Here's how the part is built. I have some questions about the finished solid (model axes, mm). Face numbers are marked on the shaded views. A direction names the side the tool comes from. Give positions to 0.01 mm unless a question says otherwise; leave off trailing zeros. Order: outer loops, then holes, each group sorted by start corner. A loop starts at its lowest first (then second) coordinate and runs counter-clockwise, first axis right, second up.
from build123d import *

# Parameters (mm, degrees)
SKETCH1_W           = 42
SKETCH1_H           = 42
BOSS_EXTRUDE1_DEPTH = 5
SKETCH2_R           = 1.65
CUT_EXTRUDE1_DEPTH  = 5
SKETCH3_W           = 5
SKETCH3_H           = 42
BOSS_EXTRUDE2_DEPTH = 10
SKETCH4_W           = 5
SKETCH4_H           = 10
BOSS_EXTRUDE3_DEPTH = 10
SKETCH5_R           = 1.65
CUT_EXTRUDE2_DEPTH  = 10
FILLET1_R           = 5
FILLET2_R           = 2
SKETCH6_R           = 11.5
CUT_EXTRUDE3_DEPTH  = 10


with BuildPart() as part:
    # Sketch1 → Boss-Extrude1 (new body)
    with BuildSketch(Plane(origin=(0, 0, 0), x_dir=(0, 0, -1), z_dir=(1, 0, 0))):
        with Locations((21, -21)):
            Rectangle(SKETCH1_W, SKETCH1_H)
    extrude(amount=BOSS_EXTRUDE1_DEPTH)

    # Sketch2 → Cut-Extrude1 (cut)
    with BuildSketch(Plane(origin=(5, 0, 0), x_dir=(0, 0, -1), z_dir=(1, 0, 0))):
        with Locations((5.5, -5.5)):
            Circle(SKETCH2_R)
        with Locations((36.5, -5.5)):
            Circle(SKETCH2_R)
        with Locations((36.5, -36.5)):
            Circle(SKETCH2_R)
        with Locations((5.5, -36.5)):
            Circle(SKETCH2_R)
    extrude(amount=-CUT_EXTRUDE1_DEPTH, mode=Mode.SUBTRACT)

    # Sketch3 → Boss-Extrude2 (add)
    with BuildSketch(Plane(origin=(0, 0, -42), x_dir=(-1, 0, 0), z_dir=(0, 0, -1))):
        with Locations((-2.5, -21)):
            Rectangle(SKETCH3_W, SKETCH3_H)
    extrude(amount=BOSS_EXTRUDE2_DEPTH)

    # Sketch4 → Boss-Extrude3 (add)
    with BuildSketch(Plane(origin=(0, 0, -52), x_dir=(-1, 0, 0), z_dir=(0, 0, -1))):
        with Locations((-2.5, -15.5)):
            Rectangle(SKETCH4_W, SKETCH4_H)
    extrude(amount=BOSS_EXTRUDE3_DEPTH)

    # Sketch5 → Cut-Extrude2 (cut)
    with BuildSketch(Plane(origin=(5, 0, 0), x_dir=(0, 0, -1), z_dir=(1, 0, 0))):
        with Locations((57, -15.5)):
            Circle(SKETCH5_R)
        with Locations((47, -32)):
            Circle(SKETCH5_R)
        with Locations((47, -12)):
            Circle(SKETCH5_R)
    extrude(amount=-CUT_EXTRUDE2_DEPTH, mode=Mode.SUBTRACT)

    # Fillet1
    fillet1_edges = [part.edges().sort_by_distance(p)[0] for p in [
        (2.5, -10.5, -62),
        (2.5, -20.5, -62),
        (2.5, -20.5, -52),
    ]]
    fillet(fillet1_edges, radius=FILLET1_R - 0.0001)  # a hair under: the kernel refuses the full size

    # Fillet2
    fillet2_edges = [part.edges().sort_by_distance(p)[0] for p in [
        (2.5, -10.5, -52),
    ]]
    fillet(fillet2_edges, radius=FILLET2_R)

    # Sketch6 → Cut-Extrude3 (cut)
    with BuildSketch(Plane(origin=(5, 0, 0), x_dir=(0, 0, -1), z_dir=(1, 0, 0))):
        with Locations((21, -21)):
            Circle(SKETCH6_R)
    extrude(amount=-CUT_EXTRUDE3_DEPTH, mode=Mode.SUBTRACT)


solid = part.part
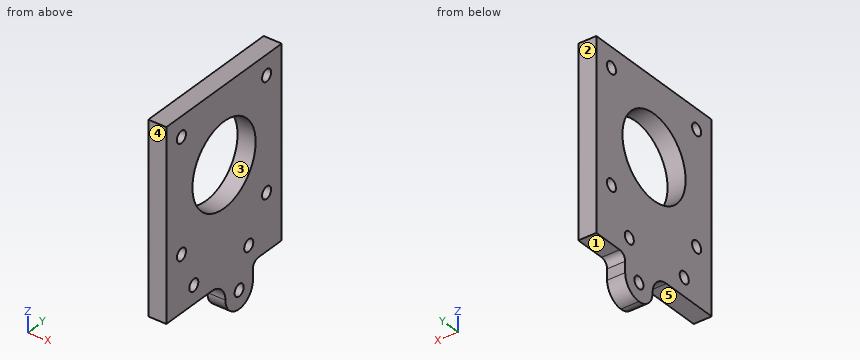
Q1. I need wall thicknesses on L1, parallel to Y at x = 2.45, z = -47; L2, parallel to Y at x = 1.8, z = -36.5; L3, parallel to Y at x = 1.35, z = -21. Which ranges of each line are inside material? Lowest first, please.
Filled sheet:
L1: y = -42 to -33.65, -30.35 to -13.65, -10.35 to 0
L2: y = -42 to -38.15, -34.85 to -7.15, -3.85 to 0
L3: y = -42 to -32.5, -9.5 to 0
Q2. If we section it at C-C on x = 1.4: Give the number of separate pieces and of enclosed holes in the cut face, plus the area to 3 significant figures.
Filled sheet:
separate pieces: 1
enclosed holes: 8
area: 1,800 mm2
Q3. For the marked faces 4 and 5, which set-ups out of +Z, -Z, +X, -X, +Y, -Y let a thin tool reach every point of the face, with its end or its side?
Filled sheet:
face 4: +Z, -Z, +X, -X, -Y
face 5: -Z, +X, -X, -Y
Q4. If we section it at B-B on z = -21: List the corners of the cut face in (x, y) for me.
Filled sheet:
outline: (0, -42) - (5, -42) - (5, -32.5) - (0, -32.5) - close; (0, -9.5) - (5, -9.5) - (5, 0) - (0, 0) - close
Q5. I'm going to push flat-ended pins straight in: P1, Ø3, axis at y = -5.5, z = -5.5, coming from the +X side; P2, Ø1.5, axis at x = 2, y = -30.5, coming from the -Z side; P3, Ø1, axis at x = 2, y = -10.5, coming from the -Z side. Where does each tip first touch, or does it pass through?
Filled sheet:
P1: passes through
P2: stops at z = -52
P3: stops at z = -59.18
Q6. If we section it at A-A on y = -5.5: List the corners of the cut face in (x, z) for me.
Filled sheet:
outline: (0, -52) - (5, -52) - (5, -38.15) - (0, -38.15) - close; (0, -34.85) - (5, -34.85) - (5, -7.15) - (0, -7.15) - close; (0, -3.85) - (5, -3.85) - (5, 0) - (0, 0) - close
Q7. Thinking about a two-plate mould opening in Y: for the marked faces 1, 2 and 3, which applies, released by +Y, released by -Y, zero draft, split by the parting line, or undercut?
Filled sheet:
face 1: zero draft
face 2: released by +Y
face 3: undercut
Q8. If we section it at D-D on z = -5.5: List the corners of the cut face in (x, y) for me.
Filled sheet:
outline: (0, -42) - (5, -42) - (5, -38.15) - (0, -38.15) - close; (0, -34.85) - (5, -34.85) - (5, -7.15) - (0, -7.15) - close; (0, -3.85) - (5, -3.85) - (5, 0) - (0, 0) - close
